Input: part model. Units: mm. Frame: model coordinates. A direction names the side the tool comes from. Give positions to 0.01 mm unless a question says otherwise; leave off trailing zeros. Loops run counter-clockwise (first coordinate to the right, second up) from the corner with the lowest first, then second, coordinate; pieces in that order, holes last. Notation, with made-up numbers: (53.25, 61) - (65.25, 61) arc R27 cw to (65.25, 77) - close; hole circle Ø7 at (20, 74). An arc over 180 degrees is marked (long way). Answer as a JSON object with one key per item and string values.
from build123d import *

# Parameters (mm, degrees)
SKIZZE1_W                            = 150
SKIZZE1_H                            = 200
AUFSATZ_LINEAR_AUSTRAGEN1_DEPTH      = 10
SKIZZE2_W                            = 70
SKIZZE2_H                            = 20
SCHNITT_LINEAR_AUSTRAGEN2_DEPTH      = 1
SCHNITT_LINEAR_AUSTRAGEN2_DEPTH_BACK = 11


with BuildPart() as part:
    # Skizze1 → Aufsatz-Linear austragen1 (new body)
    with BuildSketch(Plane(origin=(0, 0, 0), x_dir=(1, 0, 0), z_dir=(0, 1, 0))):
        with Locations((25, 50)):
            Rectangle(SKIZZE1_W, SKIZZE1_H)
    extrude(amount=AUFSATZ_LINEAR_AUSTRAGEN1_DEPTH)

    # Skizze2 → Schnitt-Linear austragen2 (cut, two sides)
    with BuildSketch(Plane.XZ) as schnitt_linear_austragen2_sk:
        with Locations((25, -50)):
            Rectangle(SKIZZE2_W, SKIZZE2_H)
    extrude(amount=SCHNITT_LINEAR_AUSTRAGEN2_DEPTH, mode=Mode.SUBTRACT)
    extrude(schnitt_linear_austragen2_sk.sketch, amount=-SCHNITT_LINEAR_AUSTRAGEN2_DEPTH_BACK, mode=Mode.SUBTRACT)


solid = part.part
Item 1: Material intervals for line 1 (X direction, y = 6.25, z = -43); line 2 (Z direction, x = 31, y = 3), sorted ascending. Write a range as [from, to].
Geometry check:
{"line 1": "x = [-50, -10], [60, 100]", "line 2": "z = [-150, -60], [-40, 50]"}
Item 2: Mould query, pull axis X, two halves, no side actions, for faces 3 (the face through (-50, 5, -49)), 4 (the face through (25, 5, -40)), 5 (the face through (24, 0, -74)). Classes: released by +X, released by -X, zero draft, split by the parting line, or undercut.
Geometry check:
{"face 3": "released by -X", "face 4": "undercut", "face 5": "zero draft"}
Item 3: Access query for faces 1 (the face through (24, 5, 50)), 2 (the face through (25, 5, -60)). Directions: +Z, -Z, +X, -X, +Y, -Y. A direction counts if a zero-diameter tool reaches every point of the face in a straight line with its end or side. Return the directions, or none.
Geometry check:
{"face 1": "+Z, +X, -X, +Y, -Y", "face 2": "+Y, -Y"}
Item 4: Cut plane C-C (y = 6.25). Return loops of the section in (x, z), then the cut area to 3 significant figures.
Geometry check:
{"outline": "(-50, -150) - (100, -150) - (100, 50) - (-50, 50) - close; hole (-10, -60) - (60, -60) - (60, -40) - (-10, -40) - close", "area": "28,600 mm2"}
Item 5: Cut plane A-A (z = -46.5). Return loops of the section in (x, y).
Geometry check:
{"outline": "(-50, 0) - (-10, 0) - (-10, 10) - (-50, 10) - close; (60, 0) - (100, 0) - (100, 10) - (60, 10) - close"}
Item 6: Cut plane B-B (x = 19). Return loops of the section in (y, z).
Geometry check:
{"outline": "(0, -150) - (10, -150) - (10, -60) - (0, -60) - close; (0, -40) - (10, -40) - (10, 50) - (0, 50) - close"}
